Autodesk Inventor part; units mm, degrees
ref_plane "YZ Plane" through (0, 0, 0) normal (1, 0, 0) x (0, 1, 0)
ref_plane "XZ Plane" through (0, 0, 0) normal (0, 1, 0) x (-1, 0, 0)
ref_plane "XY Plane" through (0, 0, 0) normal (0, 0, 1) x (1, 0, 0)
sketch "Sketch1" plane through (0, 0, 0) normal (0, 0, 1) x (1, 0, 0)
  line L0 (0, -5.5) -> (4, -5.5)
  line L1 (7, -5.5) -> (4, -5.5)
  line L2 (0, -5.5) -> (0, 0)
  line L3 (0, 0) -> (4, 0)
  line L4 (4, 5) -> (4, 0)
  line L5 (0, 5) -> (4, 5)
  line L6 (0, 5) -> (0, 10)
  line L7 (0, 10) -> (4, 10)
  line L8 (4, 15) -> (4, 10)
  line L9 (0, 15) -> (4, 15)
  line L10 (0, 15) -> (0, 20)
  line L11 (0, 20) -> (4, 20)
  line L12 (4, 25) -> (4, 20)
  line L13 (0, 25) -> (4, 25)
  line L14 (0, 25) -> (0, 30)
  line L15 (0, 30) -> (4, 30)
  line L16 (4, 32.6906) -> (4, 30)
  line L17 (7, -1.5) -> (7, -5.5)
  line L18 (7, -1.5) -> (13, -1.5)
  line L19 (13, -5.5) -> (13, -1.5)
  line L20 (17, -5.5) -> (13, -5.5)
  line L21 (17, -1.5) -> (17, -5.5)
  line L22 (17, -1.5) -> (23, -1.5)
  line L23 (23, -5.5) -> (23, -1.5)
  line L24 (27, -5.5) -> (23, -5.5)
  line L25 (27, -1.5) -> (27, -5.5)
  line L26 (27, -1.5) -> (33, -1.5)
  line L27 (33, -5.5) -> (33, -1.5)
  line L28 (37, -5.5) -> (33, -5.5)
  line L29 (37, -1.5) -> (37, -5.5)
  line L30 (37, -1.5) -> (43, -1.5)
  line L31 (43, -5.5) -> (43, -1.5)
  line L32 (47, -5.5) -> (43, -5.5)
  line L33 (47, -1.5) -> (47, -5.5)
  line L34 (47, -1.5) -> (53, -1.5)
  line L35 (53, -5.5) -> (53, -1.5)
  line L36 (57, -5.5) -> (53, -5.5)
  line L37 (57, -1.5) -> (57, -5.5)
  line L38 (57, -1.5) -> (63, -1.5)
  line L39 (63, -5.5) -> (63, -1.5)
  line L40 (67, -5.5) -> (63, -5.5)
  line L41 (67, -1.5) -> (67, -5.5)
  line L42 (67, -1.5) -> (73, -1.5)
  line L43 (73, -5.5) -> (73, -1.5)
  line L44 (77, -5.5) -> (73, -5.5)
  line L45 (77, -1.5) -> (77, -5.5)
  line L46 (77, -1.5) -> (83, -1.5)
  line L47 (83, -5.5) -> (83, -1.5)
  line L48 (87, -5.5) -> (83, -5.5)
  line L49 (87, -1.5) -> (87, -5.5)
  line L50 (87, -1.5) -> (93, -1.5)
  line L51 (93, -5.5) -> (93, -1.5)
  line L52 (97, -5.5) -> (93, -5.5)
  line L53 (97, -1.5) -> (97, -5.5)
  line L54 (97, -1.5) -> (103, -1.5)
  line L55 (103, -5.5) -> (103, -1.5)
  line L56 (107, -5.5) -> (103, -5.5)
  line L57 (107, -1.5) -> (107, -5.5)
  line L58 (107, -1.5) -> (113, -1.5)
  line L59 (113, -5.5) -> (113, -1.5)
  line L60 (117, -5.5) -> (113, -5.5)
  line L61 (117, -1.5) -> (117, -5.5)
  line L62 (117, -1.5) -> (123, -1.5)
  line L63 (123, -5.5) -> (123, -1.5)
  line L64 (126, -5.5) -> (123, -5.5)
  line L65 (126, -5.5) -> (130, -5.5)
  line L66 (130, 0) -> (130, -5.5)
  line L67 (130, 0) -> (126, 0)
  line L68 (126, 0) -> (126, 5)
  line L69 (126, 5) -> (130, 5)
  line L70 (130, 10) -> (130, 5)
  line L71 (126, 10) -> (130, 10)
  line L72 (126, 10) -> (126, 15)
  line L73 (126, 15) -> (130, 15)
  line L74 (130, 20) -> (130, 15)
  line L75 (126, 20) -> (130, 20)
  line L76 (126, 20) -> (126, 25)
  line L77 (126, 25) -> (130, 25)
  line L78 (130, 30) -> (130, 25)
  line L79 (126, 30) -> (130, 30)
  line L80 (126, 30) -> (126, 32.6906)
  line L81 (4, 32.6906) -> (126, 32.6906)
  point P0 (0, 0)
extrude "Extrusion1" add sketch "Sketch1" along normal blind 4
sketch "Sketch2" plane through (0, 0, 4) normal (0, 0, 1) x (1, 0, 0)
  line L0 (0, -5.5) -> (7, -5.5)
  line L1 (7, -5.5) -> (7, -1.5)
  line L2 (7, -1.5) -> (13, -1.5)
  line L3 (13, -1.5) -> (13, -5.5)
  line L4 (13, -5.5) -> (17, -5.5)
  line L5 (17, -5.5) -> (17, -1.5)
  line L6 (17, -1.5) -> (23, -1.5)
  line L7 (23, -1.5) -> (23, -5.5)
  line L8 (23, -5.5) -> (27, -5.5)
  line L9 (27, -5.5) -> (27, -1.5)
  line L10 (27, -1.5) -> (33, -1.5)
  line L11 (33, -1.5) -> (33, -5.5)
  line L12 (33, -5.5) -> (37, -5.5)
  line L13 (37, -5.5) -> (37, -1.5)
  line L14 (37, -1.5) -> (43, -1.5)
  line L15 (43, -1.5) -> (43, -5.5)
  line L16 (43, -5.5) -> (47, -5.5)
  line L17 (47, -5.5) -> (47, -1.5)
  line L18 (47, -1.5) -> (53, -1.5)
  line L19 (53, -1.5) -> (53, -5.5)
  line L20 (53, -5.5) -> (57, -5.5)
  line L21 (57, -5.5) -> (57, -1.5)
  line L22 (57, -1.5) -> (63, -1.5)
  line L23 (63, -1.5) -> (63, -5.5)
  line L24 (63, -5.5) -> (67, -5.5)
  line L25 (67, -5.5) -> (67, -1.5)
  line L26 (67, -1.5) -> (73, -1.5)
  line L27 (73, -1.5) -> (73, -5.5)
  line L28 (73, -5.5) -> (77, -5.5)
  line L29 (77, -5.5) -> (77, -1.5)
  line L30 (77, -1.5) -> (83, -1.5)
  line L31 (83, -1.5) -> (83, -5.5)
  line L32 (83, -5.5) -> (87, -5.5)
  line L33 (87, -5.5) -> (87, -1.5)
  line L34 (87, -1.5) -> (93, -1.5)
  line L35 (93, -1.5) -> (93, -5.5)
  line L36 (93, -5.5) -> (97, -5.5)
  line L37 (97, -5.5) -> (97, -1.5)
  line L38 (97, -1.5) -> (103, -1.5)
  line L39 (103, -1.5) -> (103, -5.5)
  line L40 (103, -5.5) -> (107, -5.5)
  line L41 (107, -5.5) -> (107, -1.5)
  line L42 (107, -1.5) -> (113, -1.5)
  line L43 (113, -1.5) -> (113, -5.5)
  line L44 (113, -5.5) -> (117, -5.5)
  line L45 (117, -5.5) -> (117, -1.5)
  line L46 (117, -1.5) -> (123, -1.5)
  line L47 (123, -1.5) -> (123, -5.5)
  line L48 (123, -5.5) -> (130, -5.5)
  line L49 (130, -5.5) -> (130, 0)
  line L50 (130, 0) -> (126, 0)
  line L51 (126, 0) -> (126, 5)
  line L52 (126, 5) -> (130, 5)
  line L53 (130, 5) -> (130, 10)
  line L54 (130, 10) -> (126, 10)
  line L55 (126, 10) -> (126, 15)
  line L56 (126, 15) -> (130, 15)
  line L57 (130, 15) -> (130, 20)
  line L58 (130, 20) -> (126, 20)
  line L59 (126, 20) -> (126, 25)
  line L60 (126, 25) -> (130, 25)
  line L61 (130, 25) -> (130, 30)
  line L62 (130, 30) -> (126, 30)
  line L63 (126, 30) -> (126, 32.6906)
  line L64 (126, 32.6906) -> (4, 32.6906)
  line L65 (4, 32.6906) -> (4, 30)
  line L66 (4, 30) -> (0, 30)
  line L67 (0, 30) -> (0, 25)
  line L68 (0, 25) -> (4, 25)
  line L69 (4, 25) -> (4, 20)
  line L70 (4, 20) -> (0, 20)
  line L71 (0, 20) -> (0, 15)
  line L72 (0, 15) -> (4, 15)
  line L73 (4, 15) -> (4, 10)
  line L74 (4, 10) -> (0, 10)
  line L75 (0, 10) -> (0, 5)
  line L76 (0, 5) -> (4, 5)
  line L77 (4, 5) -> (4, 0)
  line L78 (4, 0) -> (0, 0)
  line L79 (0, 0) -> (0, -5.5)
  point P0 (0, 0)
properties part number "VorderWand"
For this review, take the finished solid that the model builds, in its own axes (mm). A direction names the side the tool comes from. Round coordinates to 2 decimals unless told otherwise and drop trailing zeros. Order: outer loops, then holes, each group sorted by start corner. A loop starts at its lowest first (then second) coordinate and runs counter-clockwise, first axis right, second up. Notation, with made-up numbers: M 32.25,-9 L 83.25,-9 A11 ccw 83.25,3 Z; hole C 58.5,78 d10. An arc over 180 degrees is marked long. Write each question's results on one line, items separated by ' | '. Start each with the question number.
1. Draft analysis for pull direction Y (two halves, no side actions). For faces 4 (the face through (15, -5.5, 2)), 5 (the face through (4, 23, 2)), 6 (the face through (128, 5, 2)), 7 (the face through (64, 32.691, 2)), state which applies: pulls with the +Y half, pulls with the -Y half, needs draft (parallel to the pull), parting line crosses it, or undercut.
2. To check wall thickness, follow L1, parallel to X at y = 4.5, z = 2; L2, parallel to Y at x = 99.5, z = 2.3. State the ranges of each line that lie inside material, in increasing order. Write a range as [from, to].
3. Add section A-A (y = 13.5). State the section outline as (x, z) points.
4. Add section B-B (x = 119). State the section outline as (y, z) points.
5. Clearance check with flat-ended pins moving along their axes: pin 1 Ø1.5 at (y, z) = (20, 2) entering from -X; pin 2 Ø1.2 at (x, z) = (21, 2.5) entering from -Y; pin 3 Ø1.5 at (y, z) = (23, 0.5) entering from -X. State where each tip first meets the part, or that it passes through.
6. Tool access review of faces 1 (the face through (2, 25, 2)), 2 (the face through (83, -4, 2)), 3 (the face through (2, 30, 2)): name each direction out of +Z, -Z, +X, -X, +Y, -Y from which nothing blocks a thin tool from reaching the whole face with its end or side.
Output values:
1) face 4: pulls with the -Y half | face 5: undercut | face 6: undercut | face 7: pulls with the +Y half
2) L1: [4, 126] | L2: [-1.5, 32.69]
3) outline: M 4,0 L 126,0 L 126,4 L 4,4 Z
4) outline: M -1.5,0 L 32.69,0 L 32.69,4 L -1.5,4 Z
5) pin 1: x = 0 | pin 2: y = -1.5 | pin 3: x = 4
6) face 1: +Z, -Z, -X | face 2: +Z, -Z, -Y | face 3: +Z, -Z, -X, +Y
